Geometry: final body of the model. Coordinates: model frame, mm. A direction names the side the tool comes from. Round coordinates to 2 decimals unless told otherwise and drop trailing zeros. Loops run counter-clockwise (first coordinate to the right, second up) from the corner with the lowest first, then second, coordinate; pieces in that order, holes last. Notation, with made-up numbers: (11, 47.5) - (64, 47.5) arc R25 cw to (64, 84.5) - close; hole circle Ø1 at (66.25, 32.25). An arc over 180 degrees is marked (long way). Use CSV: the item, a comma, the result in double quotes.
from build123d import *

# Parameters (mm, degrees)
SKETCH1_W           = 19.05
SKETCH1_H           = 28.763083029
SKETCH1_R           = 1.5875
BOSS_EXTRUDE1_DEPTH = 0.1524
SKETCH2_W           = 0.1524
SKETCH2_H           = 28.763083029
BOSS_EXTRUDE2_DEPTH = 16.357339


with BuildPart() as part:
    # Sketch1 → Boss-Extrude1 (new body)
    with BuildSketch(Plane.XY):
        with Locations((6.35, -0.087691515)):
            Rectangle(SKETCH1_W, SKETCH1_H)
        with Locations((9.525, 0)):
            Circle(SKETCH1_R, mode=Mode.SUBTRACT)
    extrude(amount=BOSS_EXTRUDE1_DEPTH)

    # Sketch2 → Boss-Extrude2 (add)
    with BuildSketch(Plane.XY.offset(0.1524)):
        with Locations((15.7988, -0.087691515)):
            Rectangle(SKETCH2_W, SKETCH2_H)
    extrude(amount=BOSS_EXTRUDE2_DEPTH)


solid = part.part
Item 1: Section D-D on z = 6. Return the cut outline in (x, y) (3 decimals).
Final values:
outline,"(15.723, -14.469) - (15.875, -14.469) - (15.875, 14.294) - (15.723, 14.294) - close"
Item 2: Material intervals for line 1 (Z direction, x = 2.5, y = 3); line 2 (X direction, y = 0.5, z = 14.25) (3 decimals), sorted ascending.
Final values:
line 1,"z = 0 to 0.15"
line 2,"x = 15.723 to 15.875"
Item 3: Reachability of faces 1 (the flat face through (6, 0, 0.152)), 2 (the flat face through (6, 0, 0)) from +Z, -Z, +X, -X, +Y, -Y: full face, straight path, thin tool, end or side. Return the list, or none.
Final values:
face 1,"+Z, -X, +Y, -Y"
face 2,"-Z, +X, -X, +Y, -Y"
Item 4: Section B-B on x = 10.25. Return the cut outline in (y, z).
Final values:
outline,"(-14.47, 0) - (-1.41, 0) - (-1.41, 0.15) - (-14.47, 0.15) - close; (1.41, 0) - (14.29, 0) - (14.29, 0.15) - (1.41, 0.15) - close"
Item 5: Section C-C on y = -4. Return the cut outline in (x, z) (3 decimals).
Final values:
outline,"(-3.175, 0) - (15.875, 0) - (15.875, 16.51) - (15.723, 16.51) - (15.723, 0.152) - (-3.175, 0.152) - close"
Item 6: Pin query (flat end, axial travel): P1, Ø9.5, axis at x = 3.5, y = 6.5, coming from the +Z side; P2, Ø5, axis at y = -6, z = 4.5, coming from the -X side. Return the tip coordinate at first contact, or that it passes through.
Final values:
P1,"stops at z = 0.15"
P2,"stops at x = 15.72"
